Geometry: final body of the model. Coordinates: model frame, mm. Face numbers are marked on the shaded views. A direction names the side the tool comes from. Give positions to 0.01 mm unless a question says otherwise; leave off trailing zeros. Loops run counter-clockwise (first coordinate to the right, second up) from the corner with the lowest first, then second, coordinate; pieces in that order, holes last. Notation, with made-up numbers: (27, 67.25) -> (68, 67.25) arc R13 ccw to (68, 91.25) -> close; hole circle Ø7 at (-6.5, 11.25). An arc over 180 degrees is marked (long way). One line per question, with ' | ' between items. Start each with the question number.
Item 1: Section A-A on x = 10.5. Return loops of the section in (y, z) (3 decimals), then the cut area to 3 significant figures.
Item 2: Section C-C on z = 14. Return loops of the section in (x, y) (3 decimals), then the cut area to 3 significant figures.
Item 3: Pin query (flat end, axial travel): P1, Ø0.5, axis at x = -0.5, y = 16.5, coming from the -Z side; P2, Ø1, axis at x = 14, z = 14, coming from the +Y side; P3, Ø12, axis at x = 5.5, z = 11.5, coming from the -Y side. Return the tip coordinate at first contact, or that it passes through.
Item 4: Set-up query: the marked faces 1, 2 and 3. Return all of +Z, -Z, +X, -X, +Y, -Y with unobstructed straight access to the full face (end or side cutting, diameter ignored); none if empty.
Item 5: Material intervals for line 1 along X through (y, z) = (-7, 14); line 2 along X through (y, z) = (-5, -14); line 3 along Y through (x, z) = (-5, -7), sorted ascending. Write a range as [from, to].
Item 6: Section B-B on y = -6.5. Return loops of the section in (x, z).
from build123d import *

# Parameters (mm, degrees)
DODANIE_WYCI_GNI_CIE1_DEPTH     = 1.5
SZKIC1_4_W                      = 5
SZKIC1_4_H                      = 9
DODANIE_WYCI_GNI_CIE2_DEPTH     = 38
SZKIC1_5_R                      = 2
DODANIE_WYCI_GNI_CIE3_DEPTH     = 11
SZKIC2_R                        = 0.85
WYTNIJ_WYCI_GNI_CIE3_DEPTH      = 9
WYTNIJ_WYCI_GNI_CIE4_DEPTH      = 48.867724512
WYTNIJ_WYCI_GNI_CIE4_DEPTH_BACK = 10
WYTNIJ_WYCI_GNI_CIE5_DEPTH      = 10


with BuildPart() as part:
    # Szkic1 → Dodanie-wyciągnięcie1 (new body)
    with BuildSketch(Plane(origin=(0, 0, 0), x_dir=(1, 0, 0), z_dir=(0, 1, 0))):
        with BuildLine():
            Line((15.295, -19.295), (-15.295, -19.295))
            ThreePointArc((-15.295, -19.295), (-18.123427125, -18.123427125), (-19.295, -15.295))
            Line((-19.295, -15.295), (-19.295, 15.295))
            ThreePointArc((-19.295, 15.295), (-18.123427125, 18.123427125), (-15.295, 19.295))
            Line((-15.295, 19.295), (15.295, 19.295))
            ThreePointArc((15.295, 19.295), (18.123427125, 18.123427125), (19.295, 15.295))
            Line((19.295, 15.295), (19.295, -15.295))
            ThreePointArc((19.295, -15.295), (18.123427125, -18.123427125), (15.295, -19.295))
        make_face()
    extrude(amount=DODANIE_WYCI_GNI_CIE1_DEPTH)

    # Szkic1<4> → Dodanie-wyciągnięcie2 (add)
    with BuildSketch(Plane(origin=(0, 0, 0), x_dir=(1, 0, 0), z_dir=(0, 1, 0))):
        with Locations((0, -2)):
            Rectangle(SZKIC1_4_W, SZKIC1_4_H)
    extrude(amount=DODANIE_WYCI_GNI_CIE2_DEPTH)

    # Szkic1<5> → Dodanie-wyciągnięcie3 (add)
    with BuildSketch(Plane(origin=(0, 0, 0), x_dir=(1, 0, 0), z_dir=(0, 1, 0))):
        with Locations(Location((13.965358928, -13.965358928, 0), (0, 0, 270))):
            Circle(SZKIC1_5_R)
        with Locations(Location((-13.965358928, 13.965358928, 0), (0, 0, 270))):
            Circle(SZKIC1_5_R)
    extrude(amount=-DODANIE_WYCI_GNI_CIE3_DEPTH)

    # Szkic2 → Wytnij-wyciągnięcie3 (cut)
    with BuildSketch(Plane(origin=(0, -11, 0), x_dir=(1, 0, 0), z_dir=(0, 1, 0))):
        with Locations(Location((-14, 14, 0), (0, 0, 270))):
            Circle(SZKIC2_R)
        with Locations(Location((14, -14, 0), (0, 0, 270))):
            Circle(SZKIC2_R)
    extrude(amount=WYTNIJ_WYCI_GNI_CIE3_DEPTH, mode=Mode.SUBTRACT)

    # Szkic4 → Wytnij-wyciągnięcie4 (cut, two sides: drawn at the far end of the back side and taken through both)
    with BuildSketch(Plane.ZY.offset(2.5).offset(-WYTNIJ_WYCI_GNI_CIE4_DEPTH_BACK)):
        Polygon((-2.5, 5.85), (-2.5, 4), (-0.4, 4.6), (-0.4, 5.25), align=None)
        Polygon((-0.4, 2.75), (-2.5, 3.35), (-2.5, 1.5), (-0.4, 2.1), align=None)
        Polygon((-2.5, 8.35), (-2.5, 6.5), (-0.4, 7.1), (-0.4, 7.75), align=None)
        Polygon((-2.5, 10.85), (-2.5, 9), (-0.4, 9.6), (-0.4, 10.25), align=None)
        Polygon((-2.5, 13.35), (-2.5, 11.5), (-0.4, 12.1), (-0.4, 12.75), align=None)
        Polygon((-2.5, 15.85), (-2.5, 14), (-0.4, 14.6), (-0.4, 15.25), align=None)
        Polygon((-0.4, 35.25), (-2.5, 35.85), (-2.5, 34), (-0.4, 34.6), align=None)
        Polygon((-2.5, 18.35), (-2.5, 16.5), (-0.4, 17.1), (-0.4, 17.75), align=None)
        Polygon((-0.4, 32.75), (-2.5, 33.35), (-2.5, 31.5), (-0.4, 32.1), align=None)
        Polygon((-2.5, 20.85), (-2.5, 19), (-0.4, 19.6), (-0.4, 20.25), align=None)
        Polygon((-0.4, 30.25), (-2.5, 30.85), (-2.5, 29), (-0.4, 29.6), align=None)
        Polygon((-2.5, 23.35), (-2.5, 21.5), (-0.4, 22.1), (-0.4, 22.75), align=None)
        Polygon((-0.4, 27.75), (-2.5, 28.35), (-2.5, 26.5), (-0.4, 27.1), align=None)
        Polygon((-2.5, 25.85), (-2.5, 24), (-0.4, 24.6), (-0.4, 25.25), align=None)
    extrude(amount=WYTNIJ_WYCI_GNI_CIE4_DEPTH + WYTNIJ_WYCI_GNI_CIE4_DEPTH_BACK, mode=Mode.SUBTRACT)

    # Szkic4<4> → Wytnij-wyciągnięcie5 (cut)
    with BuildSketch(Plane.ZY.offset(2.5)):
        with BuildLine():
            ThreePointArc((3.5, 35), (3.236396103, 35.636396103), (2.6, 35.9))
            Line((2.6, 35.9), (2.4, 35.9))
            ThreePointArc((2.4, 35.9), (1.763603897, 35.636396103), (1.5, 35))
            Line((1.5, 35), (1.5, 1.5))
            Line((1.5, 1.5), (3.5, 1.5))
            Line((3.5, 1.5), (3.5, 35))
        make_face()
    extrude(amount=-WYTNIJ_WYCI_GNI_CIE5_DEPTH, mode=Mode.SUBTRACT)


solid = part.part
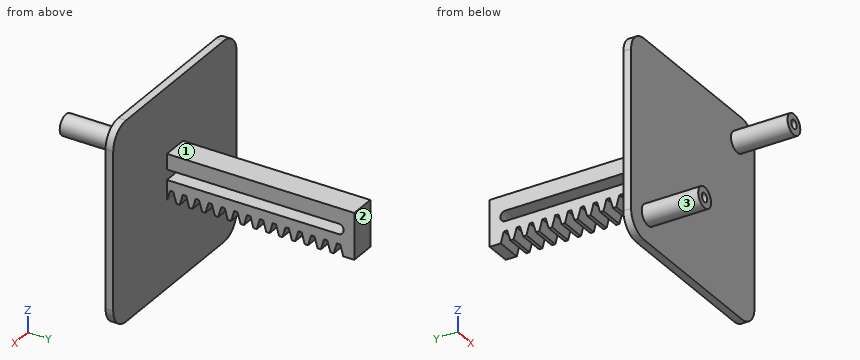
Result sheet:
1) outline: (0, -19.295) -> (1.5, -19.295) -> (1.5, 19.295) -> (0, 19.295) -> close | area: 57.9 mm²
2) outline: (-19.295, 0) -> (11.966, 0) -> (11.966, -11) -> (13.15, -11) -> (13.15, -2) -> (14.85, -2) -> (14.85, -11) -> (15.965, -11) -> (15.965, 0) -> (19.295, 0) -> (19.295, 1.5) -> (-19.295, 1.5) -> close | area: 86.6 mm²
3) P1: stops at z = -2.5 | P2: stops at y = 1.5 | P3: stops at y = 0
4) face 1: +Z, +X, -X, +Y | face 2: +Z, -Z, +X, -X, +Y | face 3: -Y
5) line 1: x = [11.97, 13.15], [14.85, 15.97] | line 2: x = [-15.97, -14.85], [-13.15, -11.97] | line 3: y = [0, 1.5]
6) outline: circle Ø4 at (-13.97, -13.97); circle Ø4 at (13.97, 13.97); hole circle Ø1.7 at (-14, -14); hole circle Ø1.7 at (14, 14)
